Can you work these out from the model? Positions are in its coordinate system, mm. Face numbers are marked on the shaded views. A direction names the side the tool comes from. Round coordinates to 2 decimals unless told otherwise and drop trailing zeros. Loops run counter-clockwise (first coordinate to the right, second up) from the corner with the lowest first, then second, coordinate; pieces in that order, holes last. Notation, with made-up numbers: (88, 52) -> (113, 52) arc R26 ccw to (113, 88) -> close; hole circle Ø9 at (24, 58.25). An arc over 180 degrees is marked (long way). Write each question's results on one line, items separated by ' | '.
from build123d import *

# Parameters (mm, degrees)
BOSS_EXTRUDE1_DEPTH  = 25
FILLET1_R            = 4.5
FILLET2_R            = 9
M5_CLEARANCE_HOLE1_D = 5.5
CUT_EXTRUDE1_DEPTH   = 5.5
CHAMFER1_SIZE        = 2


with BuildPart() as part:
    # Sketch1 → Boss-Extrude1 (new body, symmetric)
    with BuildSketch(Plane(origin=(0, 0, 0), x_dir=(0, 0, -1), z_dir=(1, 0, 0))):
        Polygon((0, 0), (-40, 0), (-40, 4.5), (-4.5, 4.5), (-4.5, 70), (0, 70), align=None)
    extrude(amount=BOSS_EXTRUDE1_DEPTH, both=True)

    # Fillet1
    fillet1_edges = [part.edges().sort_by_distance(p)[0] for p in [
        (0, 4.5, 4.5),
    ]]
    fillet(fillet1_edges, radius=FILLET1_R)

    # Fillet2
    fillet2_edges = [part.edges().sort_by_distance(p)[0] for p in [
        (0, 0, 0),
    ]]
    fillet(fillet2_edges, radius=FILLET2_R)

    # M5 Clearance Hole1 (through all)
    with Locations(Plane(origin=(0, 4.5, 0), x_dir=(-1, 0, 0), z_dir=(0, 1, 0))):
        with Locations((15, 25), (-15, 25)):
            Hole(M5_CLEARANCE_HOLE1_D / 2)

    # Sketch4 → Cut-Extrude1 (cut, through all)
    with BuildSketch(Plane.XY.offset(4.5)):
        with BuildLine():
            Line((-11.7, 60), (-11.7, 40))
            ThreePointArc((-11.7, 40), (-15, 36.7), (-18.3, 40))
            Line((-18.3, 40), (-18.3, 60))
            ThreePointArc((-18.3, 60), (-15, 63.3), (-11.7, 60))
        make_face()
        with BuildLine():
            Line((18.3, 60), (18.3, 40))
            ThreePointArc((18.3, 40), (15, 36.7), (11.7, 40))
            Line((11.7, 40), (11.7, 60))
            ThreePointArc((11.7, 60), (15, 63.3), (18.3, 60))
        make_face()
    extrude(amount=-CUT_EXTRUDE1_DEPTH, mode=Mode.SUBTRACT)

    # Chamfer1
    chamfer1_edges = [part.edges().sort_by_distance(p)[0] for p in [
        (25, 2.25, 40),
        (25, 70, 2.25),
        (-25, 70, 2.25),
        (-25, 2.25, 40),
    ]]
    chamfer(chamfer1_edges, length=CHAMFER1_SIZE)


solid = part.part
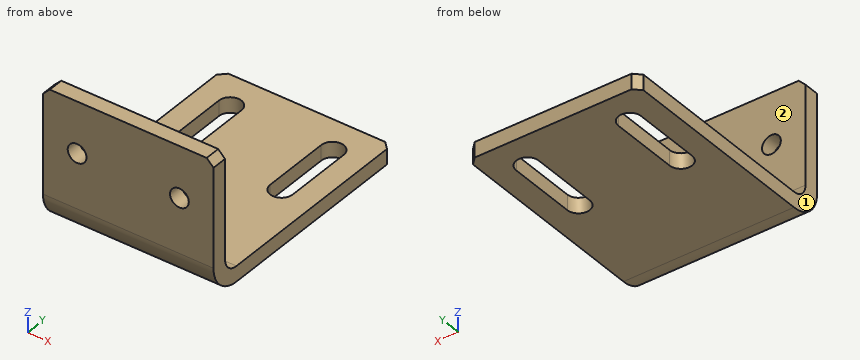
1. If we section it at C-C (z = 24): List the corners of the cut face in (x, y) for me, then the cut area to 3 significant figures.
Final values:
outline: (-25, 0) -> (-17.56, 0) -> (-17.56, 4.5) -> (-25, 4.5) -> close; (-12.44, 0) -> (12.44, 0) -> (12.44, 4.5) -> (-12.44, 4.5) -> close; (17.56, 0) -> (25, 0) -> (25, 4.5) -> (17.56, 4.5) -> close | area: 179 mm2
2. If we section it at B-B (y = 50): List the corners of the cut face in (x, z) for me, then the cut area to 3 significant figures.
Final values:
outline: (-25, 0) -> (-18.3, 0) -> (-18.3, 4.5) -> (-25, 4.5) -> close; (-11.7, 0) -> (11.7, 0) -> (11.7, 4.5) -> (-11.7, 4.5) -> close; (18.3, 0) -> (25, 0) -> (25, 4.5) -> (18.3, 4.5) -> close | area: 166 mm2
3. Please list where these lines run through material, in increasing order: line 1 (Z direction, x = 19.5, y = 52); line 2 (Y direction, x = -16, z = 2). Write a range as from..to.
Final values:
line 1: 0..4.5 | line 2: 3.34..36.86, 63.14..70
4. Will this pin go through, and if not, where does the flat tip stop? pin 1 (10 mm diameter, centred on x = -15, z = 29.5, fed in from -Y).
Final values:
pin 1: y = 0
5. If we section it at D-D (x = -22): List the corners of the cut face in (y, z) for me.
Final values:
outline: (0, 9) arc R9 ccw to (9, 0) -> (70, 0) -> (70, 4.5) -> (9, 4.5) arc R4.5 cw to (4.5, 9) -> (4.5, 40) -> (0, 40) -> close
6. If we section it at A-A (x = -15): List the corners of the cut face in (y, z) for me.
Final values:
outline: (0, 9) arc R9 ccw to (9, 0) -> (36.7, 0) -> (36.7, 4.5) -> (9, 4.5) arc R4.5 cw to (4.5, 9) -> (4.5, 22.25) -> (0, 22.25) -> close; (0, 27.75) -> (4.5, 27.75) -> (4.5, 40) -> (0, 40) -> close; (63.3, 0) -> (70, 0) -> (70, 4.5) -> (63.3, 4.5) -> close
7. On a 3-axis mill with a long thin cutter (end or side, diameter ignored), from which of +Z, -Z, +X, -X, +Y, -Y can I reach the whole of each face in a straight line? I mean the marked faces 1 and 2. Say none if no direction works.
Final values:
face 1: +Z, -Z, -X, +Y, -Y | face 2: +Z, +X, -X, +Y
